Build history of the part. All positions in model axes, mm. A direction names the side the tool comes from. Coordinates: 2 decimals unless noted, no trailing zeros. Loops run counter-clockwise (first coordinate to the right, second up) from the corner with the lowest first, then second, coordinate; pieces in that order, holes last. Notation, with made-up numbers: (89.25, 82) - (138.25, 82) arc R12 cw to (138.25, 104) - close; hole circle Ø4 at (55.5, 68.25). An arc over 180 degrees is marked (long way). One line per item, written item: value.
```python
from build123d import *

# Parameters (mm, degrees)
Y_KSEKLIK_EKSTR_ZYON1_DEPTH  = 7
Y_KSEKLIK_EKSTR_ZYON3_DEPTH  = 16
IZIM4_W                      = 28.954743141
IZIM4_H                      = 11.22646766
KES_EKSTR_ZYON1_DEPTH        = 46
IZIM5_W                      = 11.030629952
IZIM5_H                      = 8.549284238
KES_EKSTR_ZYON2_DEPTH        = 46
IZIM6_W                      = 6.045256859
IZIM6_H                      = 10.292433703
KES_EKSTR_ZYON3_DEPTH        = 46
IZIM7_W                      = 3.22646766
IZIM7_H                      = 15.019672312
KES_EKSTR_ZYON5_DEPTH        = 10
IZIM9_W                      = 11.22646766
IZIM9_H                      = 15
KES_EKSTR_ZYON6_DEPTH        = 50
KES_EKSTR_ZYON9_DEPTH        = 11.2
Y_KSEKLIK_EKSTR_ZYON4_DEPTH  = 5
Y_KSEKLIK_EKSTR_ZYON7_DEPTH  = 5
IZIM17_W                     = 17.426851058
IZIM17_H                     = 15
Y_KSEKLIK_EKSTR_ZYON8_DEPTH  = 5
Y_KSEKLIK_EKSTR_ZYON18_DEPTH = 0.028
Y_KSEKLIK_EKSTR_ZYON20_START = -10
Y_KSEKLIK_EKSTR_ZYON20_DEPTH = 20


with BuildPart() as part:
    # Çizim1 → Yükseklik-Ekstrüzyon1 (new body)
    with BuildSketch(Plane.XY):
        Polygon((42, 15), (53.195140403, 0.397642952), (82.695140403, 0.397642952), (60, 30), (8, 30), (0, 22), (0, 0), (35, 0), (35, 15), align=None)
        Polygon((61.695140403, -52.602357048), (53.195140403, -39.602357048), (53.195140403, 0.397642952), (82.695140403, 0.397642952), (82.695140403, -52.602357048), align=None)
    extrude(amount=Y_KSEKLIK_EKSTR_ZYON1_DEPTH)

    # Çizim2 → Yükseklik-Ekstrüzyon3 (add)
    with BuildSketch(Plane(origin=(0, 0, 0), x_dir=(-1, 0, 0), z_dir=(0, 0, -1))):
        Polygon((-53.195140403, 0.397642952), (-82.695140403, 0.397642952), (-60, 30), (-8, 30), (0, 22), (0, 0), (-35, 0), (-35, 15), (-42, 15), align=None)
    extrude(amount=-Y_KSEKLIK_EKSTR_ZYON3_DEPTH)

    # Çizim4 → Kes-Ekstrüzyon1 (cut)
    with BuildSketch(Plane.XZ):
        with Locations((20.522628429, 5.61323383)):
            Rectangle(IZIM4_W, IZIM4_H)
    extrude(amount=-KES_EKSTR_ZYON1_DEPTH, mode=Mode.SUBTRACT)

    # Çizim5 → Kes-Ekstrüzyon2 (cut)
    with BuildSketch(Plane(origin=(-11, 11, 0), x_dir=(0, 0, 1), z_dir=(-0.7071067811865477, 0.7071067811865475, 0))):
        with Locations((5.711152684, 19.830991305)):
            Rectangle(IZIM5_W, IZIM5_H)
    extrude(amount=-KES_EKSTR_ZYON2_DEPTH, mode=Mode.SUBTRACT)

    # Çizim6 → Kes-Ekstrüzyon3 (cut)
    with BuildSketch(Plane.XZ):
        with Locations((3.02262843, 2.853783148)):
            Rectangle(IZIM6_W, IZIM6_H)
    extrude(amount=-KES_EKSTR_ZYON3_DEPTH, mode=Mode.SUBTRACT)

    # Çizim7 → Kes-Ekstrüzyon5 (cut)
    with BuildSketch(Plane.ZY):
        with Locations((9.61323383, 14.490163844)):
            Rectangle(IZIM7_W, IZIM7_H)
    extrude(amount=-KES_EKSTR_ZYON5_DEPTH, mode=Mode.SUBTRACT)

    # Çizim9 → Kes-Ekstrüzyon6 (cut)
    with BuildSketch(Plane.ZY.offset(-35)):
        with Locations((5.61323383, 22.5)):
            Rectangle(IZIM9_W, IZIM9_H)
    extrude(amount=-KES_EKSTR_ZYON6_DEPTH, mode=Mode.SUBTRACT)

    # Çizim11 → Kes-Ekstrüzyon9 (cut)
    with BuildSketch(Plane(origin=(0, 0, 0), x_dir=(-1, 0, 0), z_dir=(0, 0, -1))):
        Polygon((-80.727385525, 2.96427975), (-71.5, 15), (-42, 15), (-51.227385525, 2.96427975), align=None)
    extrude(amount=-KES_EKSTR_ZYON9_DEPTH, mode=Mode.SUBTRACT)

    # Çizim14 → Yükseklik-Ekstrüzyon4 (add)
    with BuildSketch(Plane(origin=(82.695140403, 0, 0), x_dir=(0, 0, -1), z_dir=(1, 0, 0))):
        Polygon((-2.082581095, -49.195758149), (-2.082581095, -44.303374806), (-6.319509355, -46.749566478), align=None)
        Polygon((-2.082581095, -3.669592505), (-6.319509355, -6.115784177), (-2.082581095, -8.561975848), align=None)
    extrude(amount=Y_KSEKLIK_EKSTR_ZYON4_DEPTH)

    # Çizim15 → Yükseklik-Ekstrüzyon7 (add)
    with BuildSketch(Plane(origin=(52.274317705, 40.076976907, 0), x_dir=(0, 0, -1), z_dir=(0.7936063612919158, 0.6084315436571359, 0))):
        Polygon((-14.921026004, -44.527343425), (-11.781107025, -46.340176493), (-11.781107025, -42.714510357), align=None)
    extrude(amount=Y_KSEKLIK_EKSTR_ZYON7_DEPTH)

    # Çizim17 → Yükseklik-Ekstrüzyon8 (add)
    with BuildSketch(Plane.XY.offset(16)):
        with Locations((26.286574471, 7.5)):
            Rectangle(IZIM17_W, IZIM17_H)
    extrude(amount=Y_KSEKLIK_EKSTR_ZYON8_DEPTH)

    # Çizim21 → Yükseklik-Ekstrüzyon18 (add)
    with BuildSketch(Plane(origin=(0, 0, 11.22646766), x_dir=(-1, 0, 0), z_dir=(0, 0, -1))):
        Polygon((-42, 15), (-71.5, 15), (-60, 30), (-30.5, 30), align=None)
    extrude(amount=Y_KSEKLIK_EKSTR_ZYON18_DEPTH)

    # Çizim18 → Yükseklik-Ekstrüzyon20 (add)
    with BuildSketch(Plane(origin=(82.695140403, 0, 0), x_dir=(0, 0, -1), z_dir=(1, 0, 0)).offset(Y_KSEKLIK_EKSTR_ZYON20_START)):
        Polygon((0, 2.96427975), (-11.22646766, 26), (-11.2, 2.96427975), align=None)
    extrude(amount=-Y_KSEKLIK_EKSTR_ZYON20_DEPTH)


solid = part.part
```
Item 1: Cut at D-D, the plane z = 17. Write the cut outline in (x, y).
Check result:
outline: (17.57, 0) - (35, 0) - (35, 15) - (17.57, 15) - close
Item 2: Pull direction X, two halves, no side cores. Call faces 5 (the face through (83.32, 7.8, 13.02)), 6 (the face through (21, 15, 11.226)), 7 (the face through (26, 8, 21)): released by +X, released by -X, zero draft, split by the parting line, or undercut.
Check result:
face 5: released by +X
face 6: undercut
face 7: zero draft
Item 3: Cut at A-A, the plane z = 9.75. Write the cut outline in (x, y), then the cut area to 3 significant figures.
Check result:
outline: (0, 0) - (6.05, 0) - (6.05, 6.98) - (0, 6.98) - close; (51.23, 2.96) - (53.2, 0.4) - (82.7, 0.4) - (80.73, 2.96) - (72.7, 2.96) - (72.7, 22.97) - (52.7, 22.97) - (52.7, 2.96) - close
area: 518 mm^2
Item 4: Drop flat-ended pins along their axis: P1, Ø9, axis at x = 56.5, y = 16, coming from the +Z side; P2, Ø8, axis at x = 34.5, y = 21.5, coming from the -Z side; P3, Ø2.5, axis at x = 39, z = 13.5, coming from the -Y side; P4, Ø12, axis at x = 64.5, z = 11.5, coming from the +Y side. Give the stop position or say it passes through.
Check result:
P1: stops at z = 16
P2: stops at z = 11.2
P3: stops at y = 15
P4: stops at y = 30
Item 5: Cut at C-C, the plane x = 69. Write the cut outline in (y, z), then the cut area to 3 significant figures.
Check result:
outline: (-52.6, 0) - (2.96, 0) - (26, 11.23) - (18.26, 11.22) - (18.26, 16) - (0.4, 16) - (0.4, 7) - (-52.6, 7) - close
area: 614 mm^2
Item 6: Tool access for faces 1 (the face through (68, 0.398, 11)), 2 (the face through (85.16, -4.876, 4.171)), 3 (the face through (48, 10, 11.2)), 4 (the face through (77, 2.964, 6)): list every direction of +Z, -Z, +X, -X, +Y, -Y with a clear straight run to the whole face (end or side of a thin tool).
Check result:
face 1: +Z, +X, -Y
face 2: +Z, +X, +Y
face 3: -Z, +Y
face 4: -Z, +X, +Y
Item 7: Probe probe 1 along X at (y, z) = (5, 9.75); probe 2 along Y at (x, z) = (38, 14.5); probe 3 along Z at (x, y) = (32, 5). List the from-to ranges inside material, lowest first. Write a range as from..to.
Check result:
probe 1: x = 0..6.05, 52.7..72.7
probe 2: y = 15..30
probe 3: z = 11.23..21
